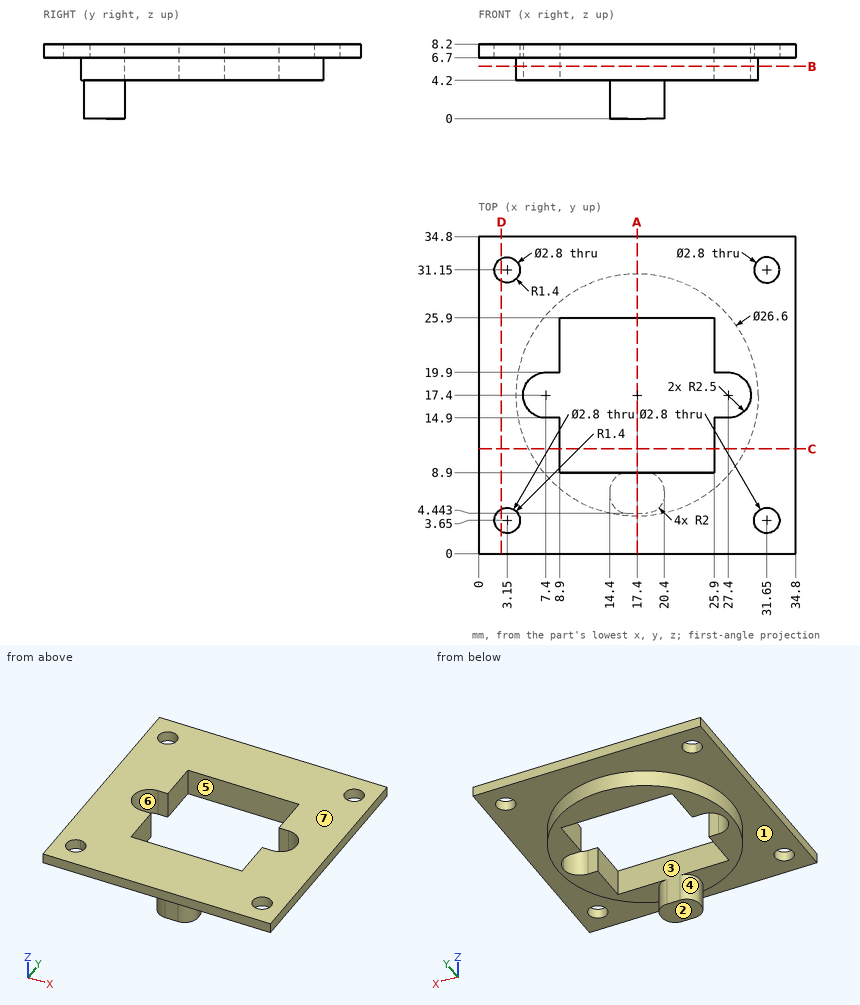
Study the drawing (mm; zero at the part's minimum x, y, z) and answer. A direction names the side the tool comes from. Coordinates: 2 decimals unless noted, no trailing zeros. Loops run counter-clockwise (first coordinate to the right, second up) from the corner with the lowest first, then second, coordinate; pieces in that order, holes last. Notation, with made-up numbers: M 45,-19 L 63,-19 A8 cw 63,-4 Z; hole C -18.5,75.25 d1. An arc over 180 degrees is marked long. Answer in a Markdown table with one row per item. Add a question column.
1. Flat-ended cylindrical pins translate along their axes: P1, Ø10, axis at x = 21.5, y = 15, coming from the -Z side; P2, Ø3.5, axis at x = 31.65, y = 3.65, coming from the -Z side; P3, Ø10.5, axis at x = 19.5, y = 15.5, coming from the -Z side; P4, Ø2, axis at y = 30, z = 5, coming from the +X side (1 decimal). Find the tip coordinate at first contact, or state that the pin passes through.
2. A tool of negligible diameter and unlimited length cuts with its end or side. For the marked faces 1, 2 and 3, from which of +Z, -Z, +X, -X, +Y, -Y can it reach the whole face along a straight path? Write none if from no direction.
3. Find section D-D, the plane x = 2.5. Write down the section's boundary in (y, z).
4. The mould has two halves that part along X. Classify the marked faces 4, 5, 6 and 7: pulls with the +X half, pulls with the -X half, needs draft (parallel to the pull), parting line crosses it, or undercut.
5. Find section B-B, the plane z = 5.75. Write down the section's boundary in (x, y), then the cut area to 3 significant figures.
6. Find section A-A, the plane x = 17.4. Write down the section's boundary in (y, z).
7. Find section C-C, the plane y = 11.5. Write down the section's boundary in (x, z).
8. Consider L1, parallel to Y at x = 3, z = 6.75; L2, parallel to Y at x = 24.5, z = 8. Determine where each line is inside the solid, lowest interval first.
Reported:
| question | item | result |
|---|---|---|
| 1 | P1 | stops at z = 4.2 |
| 1 | P2 | stops at z = 6.7 |
| 1 | P3 | passes through |
| 1 | P4 | stops at x = 23.9 |
| 2 | face 1 | -Z |
| 2 | face 2 | -Z, +X, -X, +Y, -Y |
| 2 | face 3 | +Z, -Z |
| 3 | outline | M 0,6.7 L 2.41,6.7 L 2.41,8.2 L 0,8.2 Z; M 4.89,6.7 L 29.91,6.7 L 29.91,8.2 L 4.89,8.2 Z; M 32.39,6.7 L 34.8,6.7 L 34.8,8.2 L 32.39,8.2 Z |
| 4 | face 4 | pulls with the -X half |
| 4 | face 5 | undercut |
| 4 | face 6 | undercut |
| 4 | face 7 | needs draft |
| 5 | outline | C 17.4,17.4 d26.6; hole M 7.4,14.9 L 8.9,14.9 L 8.9,8.9 L 25.9,8.9 L 25.9,14.9 L 27.4,14.9 A2.5 ccw 27.4,19.9 L 25.9,19.9 L 25.9,25.9 L 8.9,25.9 L 8.9,19.9 L 7.4,19.9 A2.5 ccw Z |
| 5 | area | 232 mm^2 |
| 6 | outline | M 0,6.7 L 4.1,6.7 L 4.1,4.2 L 4.44,4.2 L 4.44,0 L 8.9,0 L 8.9,8.2 L 0,8.2 Z; M 25.9,4.2 L 30.7,4.2 L 30.7,6.7 L 34.8,6.7 L 34.8,8.2 L 25.9,8.2 Z |
| 7 | outline | M 0,6.7 L 5.48,6.7 L 5.48,4.2 L 8.9,4.2 L 8.9,8.2 L 0,8.2 Z; M 25.9,4.2 L 29.32,4.2 L 29.32,6.7 L 34.8,6.7 L 34.8,8.2 L 25.9,8.2 Z |
| 8 | L1 | y = 0 to 2.26, 5.04 to 29.76, 32.54 to 34.8 |
| 8 | L2 | y = 0 to 8.9, 25.9 to 34.8 |
